Work out the finished part from the listing and answer in its coordinate system (mm). A direction names the side the tool comes from. Round coordinates to 2 decimals unless told otherwise and drop trailing zeros. Order: outer loops, then holes, each group sorted by start corner. A loop starts at its lowest first (then second) coordinate and runs counter-clockwise, first axis right, second up. Notation, with made-up numbers: (-27, 21.25) - (18, 21.25) arc R16 ccw to (18, 34.25) - close; hole circle Ø4 at (86.5, 27). An arc over 180 degrees is marked (long way). Use CSV: the item, a comma, the result in double quotes.
Autodesk Fusion 360 part; units mm, degrees
sketch "Sketch1" plane through (0, 0, 0) normal (0, 1, 0) x (1, 0, 0)
  circle A0 centre (0, 0) radius 7.2
  circle A1 centre (0, 0) radius 2.55
  line L0 (7.2, 0) -> (2.55, 0)
  line L1 (2.55, 0) -> (2.55, -28.2)
  line L2 (2.55, -28.2) -> (7.2, -28.2)
  line L3 (7.2, -28.2) -> (7.2, 0)
  line L4 (7.2, -28.2) -> (-3.3, -28.2)
  line L5 (-3.3, -28.2) -> (-3.3, -23.55)
  line L6 (-3.3, -23.55) -> (7.2, -23.55)
  line L7 (7.2, -23.55) -> (7.2, -28.2)
  line L8 (2.55, 0) -> (-7.2, 0)
  line L9 (7.2, -4.2775) -> (7.2, -1.15)
  line L10 (7.2, -14.1) -> (17.1595, -13.2006)
  line L11 (17.1595, -13.2006) -> (16.7494, -8.6591)
  line L12 (16.7494, -8.6591) -> (6.7899, -9.5585)
  line L13 (6.7899, -9.5585) -> (7.2, -14.1)
  line L14 (17.1595, -13.2006) -> (12.6262, -12.1654)
  line L15 (12.6262, -12.1654) -> (14.8525, -2.4164)
  line L16 (14.8525, -2.4164) -> (19.3858, -3.4516)
  line L17 (19.3858, -3.4516) -> (17.1595, -13.2006)
  dimension "d1" = 14.4
  dimension "d2" = 5.1
  dimension "d3" = 4.65
  dimension "d4" = 28.2
  dimension "d5" = 10.5
  dimension "d6" = 4.65
  dimension "d16" = 10
  dimension "d17" = 4.56
  dimension "d18" = 4.65
  dimension "d19" = 10
extrude "Extrude1" add sketch "Sketch1" along normal blind 4.65 contours A0 A1 L0 L8 | A0 L1 L3 L6 L9 L12 L13 | A0 L0 L1 | L1 L2 L3 L4 L6 L7 | L1 L4 L5 L6 | L3 L10 L12 L14 L15 | L3 L12 L13 | L11 L12 L15 L16 L17 | L11 L12 L14 L15
fillet "Fillet1" radius 2 3 edges at (14.8525, 2.325, 2.4164) (19.3858, 2.325, 3.4516) (17.1595, 2.325, 13.2006)
fillet "Fillet2" radius 2 1 edges at (7.2, 2.325, 28.2)
fillet "Fillet3" radius 2 2 edges at (-0.375, 4.65, 23.55) (-0.375, 0, 23.55)
(1) For faces 1 (the flat face through (13.875, 2.292, 6.698)), 2 (the cylindrical face through (-0.06, 2.29, -2.55)), 3 (the flat face through (-3.3, 2, 26)), 4 (the cylindrical face through (-0.33, 4.05, 24.12)), 5 (the cylindrical face through (-0.33, 0.57, 24.15)), determine the directions among +Z, -Z, +X, -X, +Y, -Y from which every point of the face is accessible in a straight line to the end or side of a thin tool.
Findings below:
face 1,"-Z, +Y, -Y"
face 2,"+Y, -Y"
face 3,"+Z, -X, +Y, -Y"
face 4,"-X, +Y"
face 5,"-X, -Y"
(2) Each of these flat-tipped pins is pushed along its axis until it touches: pin 1 (1.4 mm diameter, centred on y = 2.5, z = 6, fed in from +X); pin 2 (1 mm diameter, centred on x = 13.5, y = 3, fed in from +Z); pin 3 (1.5 mm diameter, centred on x = 15, y = 2.5, fed in from +Z). Where does it stop, or does it pass through?
Findings below:
pin 1,"stops at x = 18.96"
pin 2,"stops at z = 13.58"
pin 3,"stops at z = 13.46"
(3) Find section A-A (x = 0). Determine the outline of the cut face in (y, z), and give its area (3 significant figures).
Findings below:
outline,"(0, -7.2) - (4.65, -7.2) - (4.65, -2.55) - (0, -2.55) - close; (0, 25.55) arc R2 ccw to (2, 23.55) - (2.65, 23.55) arc R2 ccw to (4.65, 25.55) - (4.65, 28.2) - (0, 28.2) - close"
area,"41.5 mm²"
(4) Find section D-D (z = 24). Determine the outline of the cut face in (x, y), and give its area (3 significant figures).
Findings below:
outline,"(-3.3, 0.74) - (2.55, 0.74) - (2.55, 0) - (7.2, 0) - (7.2, 4.65) - (2.55, 4.65) - (2.55, 3.91) - (-3.3, 3.91) - close"
area,"40.2 mm²"
(5) Find the intervals of material crossed by L1, parallel to X at y = 3.7, z = 23; L2, parallel to X at y = 4, z = 6; L3, parallel to X at y = 2.7, z = 8.5, in increasing order. Write a range as from..to.
Findings below:
L1,"x = 2.55..7.2"
L2,"x = 2.55..7.2, 14.03..18.8"
L3,"x = 2.55..7.2, 13.46..18.23"
(6) The mould has two halves that part along X. Classify faces 6 (the flat face through (2.55, 2, 13)), 7 (the flat face through (10.32, 2.29, 9.24)), 8 (the flat face through (7.2, 2, 20)): released by +X, released by -X, zero draft, split by the parting line, or undercut.
Findings below:
face 6,"released by -X"
face 7,"undercut"
face 8,"released by +X"
(7) Find section C-C (y = 0.45). Determine the outline of the cut face in (x, z), and give its area (3 significant figures).
Findings below:
outline,"(-7.2, 0) arc R7.2 ccw to (7.2, 0) - (7.2, 9.52) - (13.36, 8.97) - (14.41, 4.37) arc R2 ccw to (16.8, 2.86) - (17.44, 3.01) arc R2 ccw to (18.94, 5.4) - (17.48, 11.78) arc R2 ccw to (15.71, 13.33) - (7.2, 14.1) - (7.2, 26.2) arc R2 ccw to (5.2, 28.2) - (-3.3, 28.2) - (-3.3, 24.29) - (2.55, 24.29) - (2.55, 0) arc R2.55 cw to (-2.55, 0) - close"
area,"298 mm²"
(8) Find section B-B (z = 3.5). Determine the outline of the cut face in (x, y).
Findings below:
outline,"(2.55, 0) - (7.2, 0) - (7.2, 4.65) - (2.55, 4.65) - close; (14.85, 0) - (18.36, 0) - (18.36, 4.65) - (14.85, 4.65) - close"
